from build123d import *

# Parameters (mm, degrees)
SKETCH2_R             = 7.5
BOSS_EXTRUDE2_DEPTH   = 14
BOSS_EXTRUDE2_2_DEPTH = 14
BOSS_EXTRUDE3_DEPTH   = 8
BOSS_EXTRUDE4_DEPTH   = 30
BOSS_EXTRUDE5_START   = 6
SKETCH6_R             = 24
SKETCH6_R_2           = 15
BOSS_EXTRUDE5_DEPTH   = 6
SKETCH7_R             = 24
SKETCH7_R_2           = 15
BOSS_EXTRUDE6_DEPTH   = 6
CUT_EXTRUDE1_REACH    = 151.907
SKETCH8_R             = 15
CUT_EXTRUDE2_REACH    = 148.253


with BuildPart() as part:
    # Sketch2 → Boss-Extrude2 (new body)
    with BuildSketch(Plane(origin=(0, 0, 0), x_dir=(1, 0, 0), z_dir=(0, 1, 0))):
        with BuildLine():
            Line((-9.632034576, 0), (11.867965424, 0))
            Line((11.867965424, 0), (11.867965424, 95))
            Line((11.867965424, 95), (-9.632034576, 95))
            ThreePointArc((-9.632034576, 95), (-20.238636294, 90.606601718), (-24.632034576, 80))
            Line((-24.632034576, 80), (-24.632034576, 15))
            ThreePointArc((-24.632034576, 15), (-20.238636294, 4.393398282), (-9.632034576, 0))
        make_face()
        with Locations(Location((-9.632034576, 15, 0), (0, 0, 270))):
            Circle(SKETCH2_R, mode=Mode.SUBTRACT)
        with Locations(Location((-9.632034576, 80, 0), (0, 0, 270))):
            Circle(SKETCH2_R, mode=Mode.SUBTRACT)
    extrude(amount=-BOSS_EXTRUDE2_DEPTH)



with BuildPart() as body_2:
    # Sketch2 → Boss-Extrude2 2 (new body)
    with BuildSketch(Plane(origin=(0, 0, 0), x_dir=(1, 0, 0), z_dir=(0, 1, 0))):
        with BuildLine():
            Line((33.867965424, 0), (55.367965424, 0))
            ThreePointArc((55.367965424, 0), (65.974567142, 4.393398282), (70.367965424, 15))
            Line((70.367965424, 15), (70.367965424, 80))
            ThreePointArc((70.367965424, 80), (65.974567142, 90.606601718), (55.367965424, 95))
            Line((55.367965424, 95), (33.867965424, 95))
            Line((33.867965424, 95), (33.867965424, 0))
        make_face()
        with Locations(Location((55.367965424, 15, 0), (0, 0, 270))):
            Circle(SKETCH2_R, mode=Mode.SUBTRACT)
        with Locations(Location((55.367965424, 80, 0), (0, 0, 270))):
            Circle(SKETCH2_R, mode=Mode.SUBTRACT)
    extrude(amount=-BOSS_EXTRUDE2_2_DEPTH)

    # Sketch4 → Boss-Extrude3 (add)
    with BuildSketch(Plane.ZY.offset(-33.867965424)):
        with BuildLine():
            ThreePointArc((-24.166847457, 71), (-48.166847457, 47), (-72.166847457, 71))
            Line((-72.166847457, 71), (-83.5, 0))
            Line((-83.5, 0), (-11.5, 0))
            Line((-11.5, 0), (-24.166847457, 71))
        make_face()
        with BuildLine():
            ThreePointArc((-24.166847457, 71), (-48.166847457, 95), (-72.166847457, 71))
            Line((-72.166847457, 71), (-24.166847457, 71))
        make_face()
        with BuildLine():
            Line((-24.166847457, 71), (-72.166847457, 71))
            ThreePointArc((-72.166847457, 71), (-48.166847457, 47), (-24.166847457, 71))
        make_face()
    extrude(amount=-BOSS_EXTRUDE3_DEPTH)


with BuildPart() as part_1:
    add(part.part)

    add(body_2.part)  # Boss-Extrude4 merges body 2
    # Sketch5 → Boss-Extrude4 (add)
    with BuildSketch(Plane.ZY.offset(-33.867965424)):
        with BuildLine():
            Line((-72.166847457, 71), (-83.5, 0))
            Line((-83.5, 0), (-11.5, 0))
            Line((-11.5, 0), (-24.166847457, 71))
            ThreePointArc((-24.166847457, 71), (-48.166847457, 47), (-72.166847457, 71))
        make_face()
        with BuildLine():
            ThreePointArc((-24.166847457, 71), (-48.166847457, 95), (-72.166847457, 71))
            ThreePointArc((-72.166847457, 71), (-48.166847457, 47), (-24.166847457, 71))
        make_face()
    extrude(amount=BOSS_EXTRUDE4_DEPTH)

    # Sketch6 → Boss-Extrude5 (add)
    with BuildSketch(Plane.ZY.offset(-3.867965424).offset(BOSS_EXTRUDE5_START)):
        with Locations((-48.166847457, 71)):
            Circle(SKETCH6_R)
        with Locations((-48.166847457, 71)):
            Circle(SKETCH6_R_2, mode=Mode.SUBTRACT)
    extrude(amount=-BOSS_EXTRUDE5_DEPTH)

    # Sketch7 → Boss-Extrude6 (add)
    with BuildSketch(Plane(origin=(41.867965424, 0, 0), x_dir=(0, 0, -1), z_dir=(1, 0, 0))):
        with Locations((48.166847457, 71)):
            Circle(SKETCH7_R)
        with Locations(Location((48.166847457, 71, 0), (0, 0, 180))):
            Circle(SKETCH7_R_2, mode=Mode.SUBTRACT)
    extrude(amount=BOSS_EXTRUDE6_DEPTH)

    # Sketch8 → Cut-Extrude1 (cut, up to next)
    with BuildSketch(Plane(origin=(41.867965424, 0, 0), x_dir=(0, 0, -1), z_dir=(1, 0, 0)), mode=Mode.PRIVATE) as cut_extrude1_sk1:
        with Locations((48.166847457, 71)):
            Circle(SKETCH8_R)
    cut_extrude1_tool1 = extrude(cut_extrude1_sk1.sketch, amount=-CUT_EXTRUDE1_REACH, mode=Mode.PRIVATE) & part_1.part
    add(cut_extrude1_tool1.solids().sort_by_distance((41.867965, 71, -48.166847))[0], mode=Mode.SUBTRACT)

    # Cut-Extrude2: up to this plane
    cut_extrude2_end = Plane(origin=(3.867965424, 12.997266696, -81.425352027), z_dir=(0, -0.1576264048748577, 0.9874988184733324))
    # Sketch9 → Cut-Extrude2 (cut, up to the surface)
    with BuildSketch(Plane(origin=(0, -1.988384564, -11.145259663), x_dir=(1, 0, 0), z_dir=(0, 0.1756331001157612, 0.9844556943528373)), mode=Mode.PRIVATE) as cut_extrude2_sk1:
        Polygon((11.867965424, 2.019780651), (11.867965424, 54.019780651), (33.588609599, 54.019780651), (33.867965424, 2.019780651), align=None)
    cut_extrude2_tool1 = split(extrude(cut_extrude2_sk1.sketch, amount=-CUT_EXTRUDE2_REACH, mode=Mode.PRIVATE), bisect_by=cut_extrude2_end, keep=Keep.BOTH, mode=Mode.PRIVATE)
    add(cut_extrude2_tool1.solids().sort_by_distance((22.798275, 25.541333, -16.056735))[0], mode=Mode.SUBTRACT)


solid = part_1.part
For this review, take the finished solid that the model builds, in its own axes (mm). A direction names the side the tool comes from. Coordinates: 2 decimals unless noted, no trailing zeros. Order: outer loops, then holes, each group sorted by start corner. A loop starts at its lowest first (then second) coordinate and runs counter-clockwise, first axis right, second up. Notation, with made-up numbers: (-30, 34.5) -> (-14, 34.5) arc R37 cw to (-14, 70.5) -> close; hole circle Ø4 at (17.25, 39.25). An arc over 180 degrees is marked (long way). Return JSON: item names as keys, results as strings.
1. We need section B-B on x = 21.5. Write out the cut boundary in (y, z).
Answer block:
{"outline": "(41.15, -76.93) -> (71, -72.17) arc R24 ccw to (71, -24.17) -> (51.19, -20.63) -> close; hole circle Ø30 at (71, -48.17)"}
2. For pin 1 Ø8 at (y, z) = (9, -32) entering from +X; pin 2 Ø17 at (x, z) = (-9.63, -15) entering from +Y; pin 3 Ø5 at (y, z) = (30.5, -62.5) entering from -X, all flat-tipped, find the tip position at first contact; note any pin that passes through.
Answer block:
{"pin 1": "x = 41.87", "pin 2": "y = 0", "pin 3": "x = 3.87"}
3. Machinability: for faces 5 (the flat face through (47.868, 55, -48)), 6 (the flat face through (35.8, 42.89, -19.15)), which of the approach directions +Z, -Z, +X, -X, +Y, -Y give a long, thin tool a straight path to every point of the face, cutting with its end or side? Answer none if there is none.
Answer block:
{"face 5": "+Z, -Z, +X, +Y", "face 6": "+Z, +X, -X, +Y"}
4. The part is to be moulded in two halves that separate along X. For faces 1 (the flat face through (-24.632, -7, -48)), 2 (the flat face through (-7, -14, -48)), 3 (the cylindrical face through (-7.379, -6.902, -72.846)), 4 (the cylindrical face through (48.046, -6.902, -16.626)), say which applies: +X half, -X half, draft (parallel to the pull), parting line (faces both ways), or undercut.
Answer block:
{"face 1": "-X half", "face 2": "draft", "face 3": "undercut", "face 4": "undercut"}
5. We need section C-C on y = 38.5. Write out the cut boundary in (x, z).
Answer block:
{"outline": "(3.87, -77.35) -> (11.87, -77.35) -> (11.87, -18.37) -> (3.87, -18.37) -> close; (33.6, -77.35) -> (41.87, -77.35) -> (41.87, -18.37) -> (33.66, -18.37) -> close"}
6. We need section A-A on y = -7. Write out the cut boundary in (x, z), and give its area (4 significant figures).
Answer block:
{"outline": "(-24.63, -80) arc R15 ccw to (-9.63, -95) -> (11.87, -95) -> (11.87, 0) -> (-9.63, 0) arc R15 ccw to (-24.63, -15) -> close; (33.87, -95) -> (55.37, -95) arc R15 ccw to (70.37, -80) -> (70.37, -15) arc R15 ccw to (55.37, 0) -> (33.87, 0) -> close; hole circle Ø15 at (-9.63, -80); hole circle Ø15 at (-9.63, -15); hole circle Ø15 at (55.37, -80); hole circle Ø15 at (55.37, -15)", "area": "6,035 mm²"}
7. For line 1 (X direction, y = -7.5, z = -15); line 2 (X direction, y = 6, z = -39.5); line 3 (Z direction, x = 1.8, y = 71), list the stretches that pass through material, from the lowest coordinate up. Write a range as from..to.
Answer block:
{"line 1": "-24.63..-17.13, -2.13..11.87, 33.87..47.87, 62.87..70.37", "line 2": "3.87..11.87, 33.81..41.87", "line 3": "-72.17..-63.17, -33.17..-24.17"}
8. We need section D-D on z = -82. Write out the cut boundary in (x, y), and give its area (3 significant figures).
Answer block:
{"outline": "(-24.5, -14) -> (-16.86, -14) -> (-16.86, 0) -> (-24.5, 0) -> close; (-2.4, -14) -> (11.87, -14) -> (11.87, 9.4) -> (3.87, 9.4) -> (3.87, 0) -> (-2.4, 0) -> close; (33.75, 9.4) -> (33.8, 0) -> (33.87, 0) -> (33.87, -14) -> (48.14, -14) -> (48.14, 0) -> (41.87, 0) -> (41.87, 9.4) -> close; (62.6, -14) -> (70.23, -14) -> (70.23, 0) -> (62.6, 0) -> close", "area": "765 mm²"}
